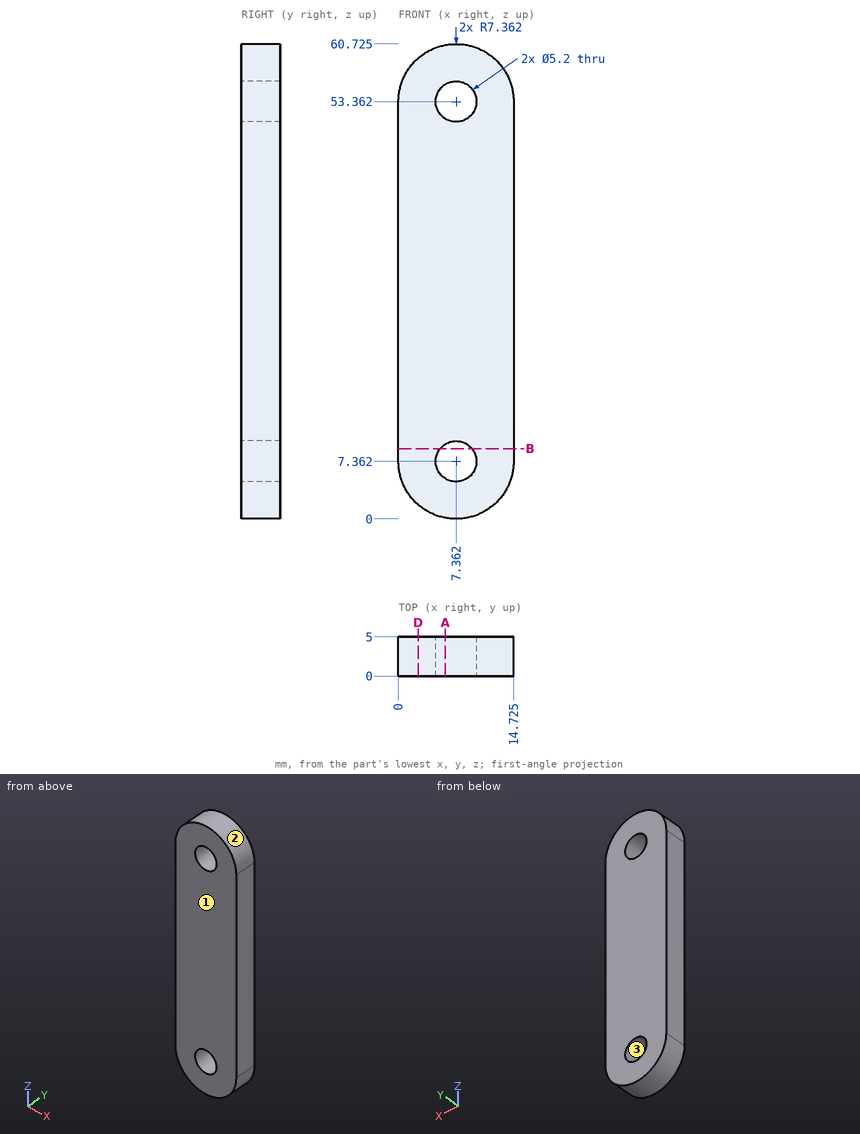
Verification items for this drawing (mm, ordinates from the low corner). Give positions to 0.01 mm unless a question says otherwise; leave off trailing zeros. Loops run counter-clockwise (first coordinate to the right, second up) from the corner with the lowest first, then second, coordinate; pieces in that order, holes last.
(1) Depth check by flat-ended pin: pin 1 Ø1 at (x, y) = (10.5, 1) entering from -Z. Enter the tip coordinate at first touch or a pass-through.
From the geometry:
pin 1: stops at z = 0.49
(2) Section check D-D on x = 2.5. Record the cut outline in (y, z) (1 decimal).
From the geometry:
outline: (0, 1.8) - (5, 1.8) - (5, 58.9) - (0, 58.9) - close
(3) Release check for a two-part mould opening along Z. For the marked faces 1, 2 and 3 record: released by +Z, released by -Z, zero draft, split by the parting line, or undercut.
From the geometry:
face 1: zero draft
face 2: released by +Z
face 3: undercut
(4) Section check A-A on x = 6. Record the cut outline in (y, z), then the cut area to 3 significant figures.
From the geometry:
outline: (0, 0.13) - (5, 0.13) - (5, 5.15) - (0, 5.15) - close; (0, 9.58) - (5, 9.58) - (5, 51.15) - (0, 51.15) - close; (0, 55.58) - (5, 55.58) - (5, 60.6) - (0, 60.6) - close
area: 258 mm2
(5) Section check B-B on z = 9. Record the cut outline in (x, y) (1 decimal).
From the geometry:
outline: (0, 0) - (5.3, 0) - (5.3, 5) - (0, 5) - close; (9.4, 0) - (14.7, 0) - (14.7, 5) - (9.4, 5) - close
(6) Thickness scan on L1, parallel to Z at x = 8.5, y = 2.15 (1 decimal); L2, parallel to Z at x = 8.75, y = 0.8 (1 decimal); L3, parallel to Z at x = 12.25, y = 1.75 (1 decimal). Record the ranges inside material, lowest first.
From the geometry:
L1: z = 0.1 to 5, 9.7 to 51, 55.7 to 60.6
L2: z = 0.1 to 5.2, 9.6 to 51.2, 55.6 to 60.6
L3: z = 1.9 to 58.9
